Can you work these out from the model? Positions are in its coordinate system, mm. Face numbers are marked on the shaded views. A direction names the side the tool comes from. Round coordinates to 2 decimals unless told otherwise and drop trailing zeros. Loops run counter-clockwise (first coordinate to the right, second up) from the corner with the lowest first, then second, coordinate; pieces in that order, holes last. Notation, with made-up numbers: (53, 48.25) -> (97, 48.25) arc R19 cw to (97, 78.25) -> close; hole circle Ø1 at (69, 51). An arc over 180 degrees is marked (long way). Answer as a JSON object with one key per item and string values.
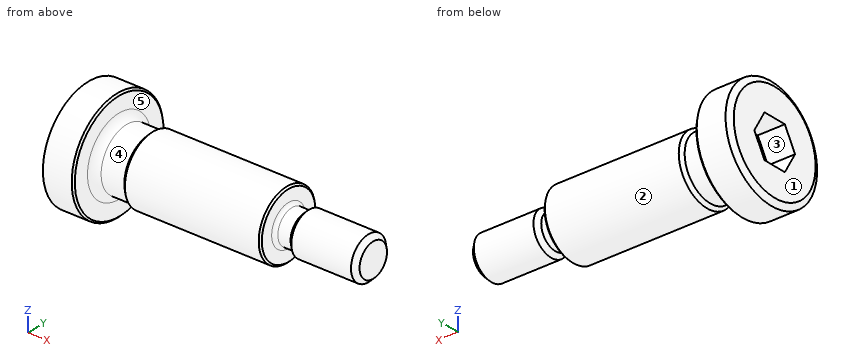
Autodesk Inventor part; units mm, degrees
ref_plane "YZ Plane" through (0, 0, 0) normal (1, 0, 0) x (0, 1, 0)
ref_plane "XZ Plane" through (0, 0, 0) normal (0, 1, 0) x (-1, 0, 0)
ref_plane "XY Plane" through (0, 0, 0) normal (0, 0, 1) x (1, 0, 0)
sketch "_____1" plane through (0, 0, 0) normal (0, 0, 1) x (1, 0, 0)
  line L0 (15, 0) -> (0.3217, 0)
  line L1 (0.3217, 0) -> (-0.4, 1.25)
  line L2 (-0.4, 1.25) -> (-2, 1.25)
  line L3 (-2, 1.25) -> (-2, 2.9036)
  line L4 (-2, 2.9036) -> (-1.8, 3.25)
  line L5 (-1.8, 3.25) -> (-0.1, 3.25)
  line L6 (-0.1, 3.25) -> (0, 3.15)
  line L7 (0, 3.15) -> (0, 2.25)
  arc A0 (0, 2.25) -> (0.44, 1.81) centre (0.44, 2.25) ccw
  line L8 (0.44, 1.81) -> (1.81, 1.81)
  line L9 (1.81, 1.81) -> (2, 2)
  line L10 (2, 2) -> (9.9, 2)
  line L11 (9.9, 2) -> (10, 1.9)
  line L12 (10, 1.9) -> (10, 1.2)
  arc A1 (10, 1.2) -> (10.2, 1) centre (10.2, 1.2) ccw
  line L13 (10.2, 1) -> (10.95, 1)
  line L14 (10.95, 1) -> (11.2, 1.25)
  line L15 (11.2, 1.25) -> (14.724, 1.25)
  line L16 (14.724, 1.25) -> (15, 0.974)
  line L17 (15, 0.974) -> (15, 0)
  line L18 (15, 0) -> (0.3217, 0)
revolve "Revolution1" add sketch "_____1" angle 360 about axis through (15, 0, 0) along (1, 0, 0)
thread "Thread1"
sketch "_____2" plane through (-2, 0, 0) normal (1, 0, 0) x (0, 0, -1)
  line L0 (-1.25, -0.7217) -> (0, -1.4434)
  line L1 (0, -1.4434) -> (1.25, -0.7217)
  line L2 (1.25, -0.7217) -> (1.25, 0.7217)
  line L3 (1.25, 0.7217) -> (0, 1.4434)
  line L4 (0, 1.4434) -> (-1.25, 0.7217)
  line L5 (-1.25, 0.7217) -> (-1.25, -0.7217)
extrude "Extrusion1" cut sketch "_____2" along normal blind 1.6
properties part number "LMSBP4-10"
Q1. I want a section at B-B, the plane x = 13.25. Write out the boundary of the cut face in (y, z), then the cut area to 3 significant figures.
Determined:
{"outline": "circle Ø2.5 at (0, 0)", "area": "4.91 mm²"}
Q2. I want a section at A-A, the plane x = 6. Write out the boundary of the cut face in (y, z).
Determined:
{"outline": "circle Ø4 at (0, 0)"}
Q3. On a 3-axis mill with a long thin cutter (end or side, diameter ignored), from which of +Z, -Z, +X, -X, +Y, -Y can I reach the whole of each face in a straight line? I mean the marked faces 1 and 2. Say none if no direction works.
Determined:
{"face 1": "+Z, -Z, -X, +Y, -Y", "face 2": "+X"}
Q4. I'm going to push flat-ended pins straight in: pin 1 (1.6 mm diameter, centred on y = 0.5, z = 0.5, fed in from -X); pin 2 (1 mm diameter, centred on y = -2.5, z = 0.5, fed in from +X). Where does each tip first touch, or does it pass through?
Determined:
{"pin 1": "x = -2", "pin 2": "x = 0.05"}
Q5. We'd pull the mould along Y, two halves only. Please class the marked faces 3, 4 and 5: pulls with the +Y half, pulls with the -Y half, needs draft (parallel to the pull), parting line crosses it, or undercut.
Determined:
{"face 3": "undercut", "face 4": "parting line crosses it", "face 5": "needs draft"}
Q6. If I drill on L1, parallel to X at y = -1.25, z = 1; L2, parallel to X at y = 2.5, z = -1; L3, parallel to Z at x = 1.5, y = 0, over which ranges is the centre line in solid material (lowest first)? Write a range as [from, to].
Determined:
{"L1": "[-2, 10]", "L2": "[-2, 0]", "L3": "[-1.81, 1.81]"}
